Verification items for the finished model (mm, model axes). Face numbers are marked on the shaded views. Coordinates: 2 decimals unless noted, no trailing zeros. Loops run counter-clockwise (first coordinate to the right, second up) from the corner with the lowest first, then second, coordinate; pieces in that order, holes last. Notation, with made-up numbers: (16.5, 19.5) -> (45.5, 19.5) arc R31 ccw to (45.5, 56.5) -> close; hole circle Ø6 at (-24, -36). An arc over 180 degrees is marked (long way). Write item = value, one per line.
```python
from build123d import *

# Parameters (mm, degrees)
F0_R     = 8.7753218572
F1_DEPTH = 6.35


with BuildPart() as f1:
    # F0 (on Front) → F1 (new body)
    with BuildSketch(Plane.XZ):
        with BuildLine():
            Line((8.7834438126, 19.115327031), (8.7753180449, 19.115327031))
            ThreePointArc((8.7753180449, 19.115327031), (8.1158254027, 22.4611173931), (6.2307064983, 25.3028722046))
            ThreePointArc((6.2307064983, 25.3028722046), (-4.4505028044, 26.673563518), (-8.4172791945, 16.6619846257))
            ThreePointArc((-8.4172791945, 16.6619846257), (-8.3844908458, 16.547589737), (-8.3526665154, 16.4329229223))
            ThreePointArc((-8.3526665154, 16.4329229223), (-9.8106463605, 5.532295474), (-18.6392198096, -1.0255757391))
            ThreePointArc((-18.6392198096, -1.0255757391), (-24.1599350394, -13.9350611847), (-10.2210623661, -15.6205699261))
            ThreePointArc((-10.2210623661, -15.6205699261), (-0.0047850834, -11.2618653325), (10.2077845484, -15.6292499923))
            ThreePointArc((10.2077845484, -15.6292499923), (24.148084509, -13.9555869055), (18.6383415606, -1.0414146996))
            ThreePointArc((18.6383415606, -1.0414146996), (17.5809373703, -0.7383140879), (16.5502978295, -0.3539240006))
            ThreePointArc((16.5502978295, -0.3539240006), (9.2433481318, 6.600298379), (8.4314352612, 16.6548257314))
            ThreePointArc((8.4314352612, 16.6548257314), (8.6949959346, 17.8725502343), (8.7834438126, 19.115327031))
        make_face()
        with BuildLine():
            ThreePointArc((-19.6872001667, -3.3644723848), (-12.9274465593, -3.6452218097), (-9.6260458218, -9.5506296907))
            ThreePointArc((-9.6260458218, -9.5506296907), (-20.189393023, -15.4560375718), (-19.6872001667, -3.3644723848))
        make_face(mode=Mode.SUBTRACT)
        with Locations((-0.0637440243, -0.0636884644)):
            Circle(F0_R, mode=Mode.SUBTRACT)
        with BuildLine():
            ThreePointArc((12.7573186389, -15.3673792813), (13.2515512011, -3.4674783406), (23.4826717993, -9.5646973403))
            ThreePointArc((23.4826717993, -9.5646973403), (19.8490444587, -15.6619163401), (12.7573186389, -15.3673792813))
        make_face(mode=Mode.SUBTRACT)
        with BuildLine():
            Line((-6.9544768432, 13.7717279244), (-6.9544670424, 13.7741073238))
            ThreePointArc((-6.9544670424, 13.7741073238), (-6.943095823, 13.7593168639), (-6.9316931846, 13.7445506127))
            Line((-6.9316931846, 13.7445506127), (-6.9316934696, 13.7422512771))
            ThreePointArc((-6.9316934696, 13.7422512771), (-6.9431007991, 13.75697751), (-6.9544768432, 13.7717279244))
        make_face(mode=Mode.SUBTRACT)
        with BuildLine():
            ThreePointArc((6.9298815278, 18.7318516666), (2.4688362723, 12.6343784947), (-4.9148938035, 14.2345766142))
            ThreePointArc((-4.9148938035, 14.2345766142), (-4.884841452, 24.0424621937), (4.9230157544, 24.0042561422))
            ThreePointArc((4.9230157544, 24.0042561422), (6.4163077672, 21.7597482397), (6.9404959307, 19.115327031))
            ThreePointArc((6.9404959307, 19.115327031), (6.9378418219, 18.9235159126), (6.9298815278, 18.7318516666))
        make_face(mode=Mode.SUBTRACT)
        with BuildLine():
            ThreePointArc((6.2307064983, 25.3028722046), (8.1158254027, 22.4611173931), (8.7753180449, 19.115327031))
            Line((8.7753180449, 19.115327031), (8.7834438126, 19.115327031))
            ThreePointArc((8.7834438126, 19.115327031), (8.1201949286, 22.4620486758), (6.2307064983, 25.3028722046))
        make_face()
        with BuildLine():
            ThreePointArc((-8.4172791945, 16.6619846257), (-4.4505028044, 26.673563518), (6.2307064983, 25.3028722046))
            ThreePointArc((6.2307064983, 25.3028722046), (-4.5601182711, 26.6209449467), (-8.3526665154, 16.4329229223))
            ThreePointArc((-8.3526665154, 16.4329229223), (-8.3844908458, 16.547589737), (-8.4172791945, 16.6619846257))
        make_face()
    extrude(amount=F1_DEPTH)


solid = f1.part
```
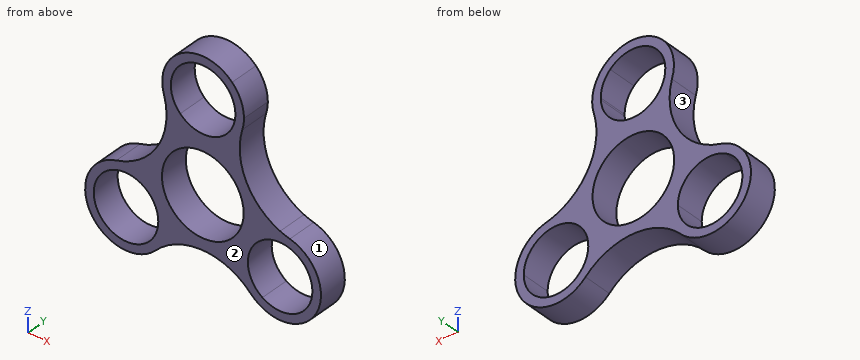
1) Sectioned sample at C-C, the plane x = 18. Record the cut outline in (y, z), plus the area to 3 significant figures.
Ans:
outline = (-6.35, -18.22) -> (0, -18.22) -> (0, -16.34) -> (-6.35, -16.34) -> close; (-6.35, -2.79) -> (0, -2.79) -> (0, -0.87) -> (-6.35, -0.87) -> close
area = 24.1 mm2
2) Material ranges on line 1 (Z direction, x = -3, y = -5.5); line 2 (X direction, y = -1.25, z = -8) (3 decimals); line 3 (X direction, y = -4.5, z = -10), recorded low to high.
Ans:
line_1 = -11.58 to -8.33, 8.21 to 12.87, 25.37 to 27.37
line_2 = -25.196 to -23.315, -9.802 to -3.808, 3.681 to 9.797, 23.304 to 25.185
line_3 = -25.32 to -23.48, -9.64 to 9.63, 23.47 to 25.31
3) Sectioned sample at A-A, the plane z = -2. Record the cut outline in (x, y).
Ans:
outline = (-21.03, -6.35) -> (-8.62, -6.35) -> (-8.62, 0) -> (-21.03, 0) -> close; (8.5, -6.35) -> (21, -6.35) -> (21, 0) -> (8.5, 0) -> close
4) Depth check by flat-ended pin: pin 1 Ø2 at (x, y) = (3.5, -3) entering from +Z. Enter the tip coordinate at first touch or a pass-through.
Ans:
pin_1 = 27.54
5) Sectioned sample at B-B, the plane x = 0. Record the cut outline in (y, z).
Ans:
outline = (-6.35, -11.26) -> (0, -11.26) -> (0, -8.84) -> (-6.35, -8.84) -> close; (-6.35, 8.71) -> (0, 8.71) -> (0, 12.18) -> (-6.35, 12.18) -> close; (-6.35, 26.06) -> (0, 26.06) -> (0, 27.9) -> (-6.35, 27.9) -> close
6) Release check for a two-part mould opening along X. For the marked faces 1, 2 and 3 record: pulls with the +X half, pulls with the -X half, needs draft (parallel to the pull), parting line crosses it, or undercut.
Ans:
face_1 = undercut
face_2 = needs draft
face_3 = pulls with the -X half
